```python
from build123d import *

# Parameters (mm, degrees)
CUT_EXTRUDE1_DEPTH  = 31.5
SKETCH3_R           = 6
CUT_EXTRUDE2_DEPTH  = 31.5
SKETCH4_R           = 7.5
SKETCH4_R_2         = 6
BOSS_EXTRUDE1_DEPTH = 13


with BuildPart() as part:
    # Sketch1 → Revolve1 (revolve)
    with BuildSketch(Plane.XY):
        Polygon((23, 0), (25, 0), (25, 40), (22, 40), (22, 43), (25, 43), (25, 46.5), (22, 46.5), (22, 49.5), (25, 49.5), (25, 57.5), (0, 57.5), (0, 56.203662834), (23, 56.203662834), (23, 51.5), (20, 51.5), (20, 44.75), (20, 38), (23, 38), align=None)
    revolve(axis=Axis((0, 63, 0), (0, -1, 0)))

    # Sketch2 → Cut-Extrude1 (cut, symmetric)
    with BuildSketch(Plane.XY):
        with BuildLine():
            Line((-17.5, 0), (17.5, 0))
            ThreePointArc((17.5, 0), (0, 10), (-17.5, 0))
        make_face()
    extrude(amount=CUT_EXTRUDE1_DEPTH, both=True, mode=Mode.SUBTRACT)

    # Sketch3 → Cut-Extrude2 (cut, symmetric)
    with BuildSketch(Plane.XY):
        with Locations((0, 30)):
            Circle(SKETCH3_R)
    extrude(amount=CUT_EXTRUDE2_DEPTH, both=True, mode=Mode.SUBTRACT)

    # Sketch4 → Boss-Extrude1 (add)
    with BuildSketch(Plane.XY.offset(10)):
        with Locations((0, 30)):
            Circle(SKETCH4_R)
        with Locations((0, 30)):
            Circle(SKETCH4_R_2, mode=Mode.SUBTRACT)
    boss_extrude1 = extrude(amount=BOSS_EXTRUDE1_DEPTH)

    # Mirror1: Boss-Extrude1 across plane
    add(boss_extrude1.mirror(Plane.XY))


solid = part.part
```
Read the model definition and answer for the solid it produces. Units are mm, in the model's axes. A direction names the side the tool comes from. Give positions to 0.01 mm unless a question says otherwise; leave off trailing zeros. Write each loop counter-clockwise with the first axis right and the second up, starting at its lowest first coordinate (ties: lowest second). Pieces come first, ordered by that corner, then holes. Notation, with made-up numbers: (25.5, 23) - (47.5, 23) arc R22 cw to (47.5, 39) - close; hole circle Ø3 at (58.5, -10). An arc over 180 degrees is marked (long way). Write item = value, one per line. Start each with the question number.
Item 1: Find section A-A (y = 30). Give the vertices of the cut face in (x, z).
Item 2: Find the intervals of material crossed by probe 1 along Y at (x, z) = (-22.5, -0.5); probe 2 along Y at (x, z) = (0, -21); probe 3 along Y at (x, z) = (0, 14), in increasing order. Write a range as [from, to].
Item 3: A tool of negligible diameter and unlimited length cuts with its end or side. For faces 4 (the flat face through (1.7, 40, -22.1)), 5 (the flat face through (2, 36, -10)), 6 (the flat face through (23.2, 0, 0.1)), from which of +Z, -Z, +X, -X, +Y, -Y can it reach the whole face along a straight path? Write none if from no direction.
Item 4: Each of these flat-tipped pins is pushed along its axis until it touches: P1, Ø16.5, axis at x = -3, y = 29, coming from the +Z side; P2, Ø1, axis at y = 28, z = 11.5, coming from the +X side; P3, Ø5, axis at y = 24, z = -16, coming from the -X side; P4, Ø5, axis at x = -13, z = 12, coming from the -Y side. Where does it stop, or does it pass through?
Item 5: The mould has two halves that part along X. Classify faces 1 (the flat face through (7, 38, 19)), 2 (the flat face through (-1.7, 49.5, -22.1)), 3 (the cylindrical face through (23.846, 44.774, 7.509)): +X half, -X half, draft (parallel to the pull), parting line (faces both ways), or undercut.
Item 6: Find section D-D (y = 47.5). Give the vertices of the cut face in (x, z), then the cut area to 3 significant figures.
Item 7: Find section C-C (x = 0). State how many separate pieces and enclosed holes the cut face has, then the cut area to 3 significant figures.
Response:
q1.outline = (-7.5, -21.74) arc R23 cw to (-7.5, 21.74) - (-7.5, 10) - (-6, 10) - (-6, 24.27) arc R25 ccw to (-6, -24.27) - (-6, -10) - (-7.5, -10) - close; (6, -24.27) arc R25 ccw to (6, 24.27) - (6, 10) - (7.5, 10) - (7.5, 21.74) arc R23 cw to (7.5, -21.74) - (7.5, -10) - (6, -10) - close
q2.probe_1 = [38, 40], [43, 46.5], [49.5, 51.5], [56.2, 57.5]
q2.probe_2 = [22.5, 24], [36, 37.5], [38, 51.5], [56.2, 57.5]
q2.probe_3 = [22.5, 24], [36, 37.5], [56.2, 57.5]
q3.face_4 = none
q3.face_5 = -Y
q3.face_6 = +Z, -Z, +X, -X, -Y
q4.P1 = 25
q4.P2 = 22.45
q4.P3 = -21.04
q4.P4 = 38
q5.face_1 = undercut
q5.face_2 = draft
q5.face_3 = parting line
q6.outline = circle Ø44 at (0, 0); hole circle Ø40 at (0, 0)
q6.area = 264 mm²
q7.separate_pieces = 3
q7.enclosed_holes = 0
q7.area = 325 mm²
